Build history of the part. All positions in model axes, mm. A direction names the side the tool comes from. Round coordinates to 2 decimals unless told otherwise and drop trailing zeros. Loops run counter-clockwise (first coordinate to the right, second up) from the corner with the lowest first, then second, coordinate; pieces in that order, holes last. Notation, with made-up numbers: (-12.75, -8) - (14.25, -8) arc R28 cw to (14.25, 24) - close; hole circle Ø2 at (66.5, 82). An arc over 180 degrees is marked (long way). Use one line per item in the form item = value. Start each with the question number.
Q1. Mould opens along X. For faces 1 (the face through (30.35, 1.9, 4.93)), 2 (the face through (-7, 7, 0)), 3 (the face through (61.05, 32.78, 1.48)) say: released by +X, released by -X, zero draft, split by the parting line, or undercut.
Q2. Pin check, flat tips, straight feed: pin 1 (4 mm diameter, centred on x = 55.5, y = 19, fed in from +Z); pin 2 (4 mm diameter, centred on x = 27.25, y = 0.92, fed in from -Z); pin 3 (3.5 mm diameter, centred on y = -14, z = 6, fed in from -X); pin 4 (2.5 mm diameter, centred on x = -73, z = 7, fed in from -Y). Stop position of each tip, or through.
Q3. Saw through at D-D (x = 4). Give the cut face in (y, z).
Q4. Saw through at A-A (x = -30). Give the cut face in (y, z), then the cut area to 3 significant figures.
Q5. 3-axis set-ups, long thin cutter, end or side, ignore diameter. For faces 4 (the face through (-68.8, -4.076, 6.549)), 5 (the face through (-9, 33.922, 5)), 6 (the face through (51.2, 32.924, 6.451)): which of +Z, -Z, +X, -X, +Y, -Y reach the whole face in a straight line?
Q6. Drill centre lines: line 1 (Y direction, x = 27, z = 3); line 2 (Y direction, x = 5, z = 7.5); line 3 (X direction, y = 8, z = 1.75). Where is each one in solid material? Low to high.
Q7. Saw through at C-C (z = 1.5). Give the cut face in (x, y).
Q8. Saw through at B-B (z = 8.25). Give the cut face in (x, y), then the cut area to 3 significant figures.
```python
from build123d import *

# Parameters (mm, degrees)
SKETCH1_R           = 5
SKETCH1_R_2         = 3.25
BOSS_EXTRUDE1_DEPTH = 10
CUT_EXTRUDE1_DEPTH  = 7
SKETCH3_R           = 2.5
CUT_EXTRUDE2_DEPTH  = 10
FILLET1_R           = 3.5


with BuildPart() as part:
    # Sketch1 → Boss-Extrude1 (new body)
    with BuildSketch(Plane.XY):
        with BuildLine():
            Line((-73.747603834, 33.92172524), (58.252396166, 33.92172524))
            ThreePointArc((58.252396166, 33.92172524), (61.080823291, 32.750152364), (62.252396166, 29.92172524))
            Line((62.252396166, 29.92172524), (62.252396166, -17.07827476))
            ThreePointArc((62.252396166, -17.07827476), (61.080823291, -19.906701885), (58.252396166, -21.07827476))
            Line((58.252396166, -21.07827476), (-73.747603834, -21.07827476))
            ThreePointArc((-73.747603834, -21.07827476), (-76.576030959, -19.906701885), (-77.747603834, -17.07827476))
            Line((-77.747603834, -17.07827476), (-77.747603834, 29.92172524))
            ThreePointArc((-77.747603834, 29.92172524), (-76.576030959, 32.750152364), (-73.747603834, 33.92172524))
        make_face()
        with Locations((-29.747603834, 3.92172524)):
            Circle(SKETCH1_R, mode=Mode.SUBTRACT)
        with Locations((2.252396166, 5.92172524)):
            Circle(SKETCH1_R_2, mode=Mode.SUBTRACT)
        with Locations((27.252396166, 0.92172524)):
            Circle(SKETCH1_R_2, mode=Mode.SUBTRACT)
    extrude(amount=BOSS_EXTRUDE1_DEPTH)

    # Sketch2 → Cut-Extrude1 (cut)
    with BuildSketch(Plane.XY.offset(10)):
        with BuildLine():
            Line((-77.747603834, -3.07827476), (-71.247603834, -3.07827476))
            ThreePointArc((-71.247603834, -3.07827476), (-68.7727301, -4.103401026), (-67.747603834, -6.57827476))
            Line((-67.747603834, -6.57827476), (-67.747603834, -21.07827476))
            Line((-67.747603834, -21.07827476), (-77.747603834, -21.07827476))
            Line((-77.747603834, -21.07827476), (-77.747603834, -3.07827476))
        make_face()
        with BuildLine():
            Line((62.252396166, 15.92172524), (55.752396166, 15.92172524))
            ThreePointArc((55.752396166, 15.92172524), (53.277522432, 16.946851505), (52.252396166, 19.42172524))
            Line((52.252396166, 19.42172524), (52.252396166, 33.92172524))
            Line((52.252396166, 33.92172524), (62.252396166, 33.92172524))
            Line((62.252396166, 33.92172524), (62.252396166, 15.92172524))
        make_face()
    extrude(amount=-CUT_EXTRUDE1_DEPTH, mode=Mode.SUBTRACT)

    # Sketch3 → Cut-Extrude2 (cut)
    with BuildSketch(Plane.XY.offset(3)):
        with Locations((-72.747603834, -8.07827476)):
            Circle(SKETCH3_R)
        with Locations((57.252396166, 20.92172524)):
            Circle(SKETCH3_R)
    extrude(amount=-CUT_EXTRUDE2_DEPTH, mode=Mode.SUBTRACT)

    # Fillet1
    fillet1_edges = [part.edges().sort_by_distance(p)[0] for p in [
        (-67.747603834, -21.07827476, 6.5),
        (-77.747603834, -3.07827476, 6.5),
        (52.252396166, 33.92172524, 6.5),
        (62.252396166, 15.92172524, 6.5),
    ]]
    fillet(fillet1_edges, radius=FILLET1_R)


solid = part.part
```
Report:
q1.face_1 = undercut
q1.face_2 = zero draft
q1.face_3 = released by +X
q2.pin_1 = 3
q2.pin_2 = through
q2.pin_3 = -67.75
q2.pin_4 = -3.08
q3.outline = (-21.08, 0) - (3.18, 0) - (3.18, 10) - (-21.08, 10) - close; (8.66, 0) - (33.92, 0) - (33.92, 10) - (8.66, 10) - close
q4.outline = (-21.08, 0) - (-1.07, 0) - (-1.07, 10) - (-21.08, 10) - close; (8.92, 0) - (33.92, 0) - (33.92, 10) - (8.92, 10) - close
q4.area = 450 mm²
q5.face_4 = +Z, -X, -Y
q5.face_5 = +Z, -Z, +X, -X, +Y
q5.face_6 = +Z, +X, +Y
q6.line_1 = -21.08 to -2.32, 4.16 to 33.92
q6.line_2 = -21.08 to 4.19, 7.66 to 33.92
q6.line_3 = -77.75 to -32.64, -26.85 to -0.25, 4.75 to 62.25
q7.outline = (-77.75, -17.08) arc R4 ccw to (-73.75, -21.08) - (58.25, -21.08) arc R4 ccw to (62.25, -17.08) - (62.25, 29.92) arc R4 ccw to (58.25, 33.92) - (-73.75, 33.92) arc R4 ccw to (-77.75, 29.92) - close; hole circle Ø5 at (-72.75, -8.08); hole circle Ø10 at (-29.75, 3.92); hole circle Ø6.5 at (2.25, 5.92); hole circle Ø6.5 at (27.25, 0.92); hole circle Ø5 at (57.25, 20.92)
q8.outline = (-77.75, 0.42) arc R3.5 ccw to (-74.25, -3.08) - (-71.25, -3.08) arc R3.5 cw to (-67.75, -6.58) - (-67.75, -17.58) arc R3.5 ccw to (-64.25, -21.08) - (58.25, -21.08) arc R4 ccw to (62.25, -17.08) - (62.25, 12.42) arc R3.5 ccw to (58.75, 15.92) - (55.75, 15.92) arc R3.5 cw to (52.25, 19.42) - (52.25, 30.42) arc R3.5 ccw to (48.75, 33.92) - (-73.75, 33.92) arc R4 ccw to (-77.75, 29.92) - close; hole circle Ø10 at (-29.75, 3.92); hole circle Ø6.5 at (2.25, 5.92); hole circle Ø6.5 at (27.25, 0.92)
q8.area = 7,180 mm²
